Geometry check sheet. Reference: the model listing, model coordinates, mm. Give positions to 0.01 mm unless a question says otherwise; leave off trailing zeros. Loops run counter-clockwise (first coordinate to the right, second up) from the corner with the lowest first, then second, coordinate; pieces in that order, holes last. Notation, with made-up numbers: (79.5, -5.75) -> (117.5, -5.75) arc R35 ccw to (117.5, 26.25) -> close; hole circle Ø10 at (-1.75, -34). An arc over 180 degrees is marked (long way). Write item = value, one per line. Start each with the question number.
```python
from build123d import *

# Parameters (mm, degrees)
F1_DEPTH = 10


# Not quite as in the source:
# - a feature names something its author has since deleted; it is built from what else it names


with BuildPart() as f1:
    # F0 (on Front) → F1 (new body)
    with BuildSketch(Plane.XZ):
        with BuildLine():
            Line((-0.4689496755, 31.1130427234), (-12.4689496755, 31.1130427234))
            Line((-12.4689496755, 31.1130427234), (-12.4689496755, 20.1130427234))
            Line((-12.4689496755, 20.1130427234), (-6.4189496755, 20.1130427234))
            ThreePointArc((-6.4189496755, 20.1130427234), (-4.9689496755, 21.5630427234), (-3.5189496755, 20.1130427234))
            ThreePointArc((-3.5189496755, 20.1130427234), (-3.9436448428, 19.0877378907), (-4.9689496755, 18.6630427234))
            Line((-4.9689496755, 18.6630427234), (-4.9689496755, 13.4656252339))
            Line((-4.9689496755, 13.4656252339), (-0.4689496755, 13.4656252339))
            Line((-0.4689496755, 13.4656252339), (-0.4689496755, 31.1130427234))
        make_face()
        with BuildLine():
            Line((-12.4689496755, 31.1130427234), (-24.4689496755, 31.1130427234))
            Line((-24.4689496755, 31.1130427234), (-24.4689496755, 20.1130427234))
            Line((-24.4689496755, 20.1130427234), (-21.4189496755, 20.1130427234))
            ThreePointArc((-21.4189496755, 20.1130427234), (-19.9689496755, 21.5630427234), (-18.5189496755, 20.1130427234))
            Line((-18.5189496755, 20.1130427234), (-12.4689496755, 20.1130427234))
            Line((-12.4689496755, 20.1130427234), (-12.4689496755, 31.1130427234))
        make_face()
        with BuildLine():
            Line((-6.4189496755, 20.1130427234), (-12.4689496755, 20.1130427234))
            Line((-12.4689496755, 20.1130427234), (-18.5189496755, 20.1130427234))
            ThreePointArc((-18.5189496755, 20.1130427234), (-18.9436448428, 19.0877378907), (-19.9689496755, 18.6630427234))
            Line((-19.9689496755, 18.6630427234), (-19.9689496755, 6.5630427234))
            ThreePointArc((-19.9689496755, 6.5630427234), (-18.9436448428, 6.1383475561), (-18.5189496755, 5.1130427234))
            Line((-18.5189496755, 5.1130427234), (-6.4189496755, 5.1130427234))
            ThreePointArc((-6.4189496755, 5.1130427234), (-5.9942545082, 6.1383475561), (-4.9689496755, 6.5630427234))
            Line((-4.9689496755, 6.5630427234), (-4.9689496755, 13.4656252339))
            Line((-4.9689496755, 13.4656252339), (-4.9689496755, 18.6630427234))
            ThreePointArc((-4.9689496755, 18.6630427234), (-5.9942545082, 19.0877378907), (-6.4189496755, 20.1130427234))
        make_face()
        with BuildLine():
            Line((-21.4189496755, 20.1130427234), (-24.4689496755, 20.1130427234))
            Line((-24.4689496755, 20.1130427234), (-24.4689496755, -0.8869572766))
            Line((-24.4689496755, -0.8869572766), (-0.4689496755, -0.8869572766))
            Line((-0.4689496755, -0.8869572766), (-0.4689496755, 13.4656252339))
            Line((-0.4689496755, 13.4656252339), (-4.9689496755, 13.4656252339))
            Line((-4.9689496755, 13.4656252339), (-4.9689496755, 6.5630427234))
            ThreePointArc((-4.9689496755, 6.5630427234), (-3.9436448428, 6.1383475561), (-3.5189496755, 5.1130427234))
            ThreePointArc((-3.5189496755, 5.1130427234), (-4.9689496755, 3.6630427234), (-6.4189496755, 5.1130427234))
            Line((-6.4189496755, 5.1130427234), (-18.5189496755, 5.1130427234))
            ThreePointArc((-18.5189496755, 5.1130427234), (-20.9942545082, 4.0877378907), (-19.9689496755, 6.5630427234))
            Line((-19.9689496755, 6.5630427234), (-19.9689496755, 18.6630427234))
            ThreePointArc((-19.9689496755, 18.6630427234), (-20.9942545082, 19.0877378907), (-21.4189496755, 20.1130427234))
        make_face()
    extrude(amount=F1_DEPTH)


solid = f1.part
```
1) Section check B-B (z = 19.5). Enter the section's corners in (x, y), plus the area to 3 significant figures.
2) Thickness scan on line 1 (X direction, y = -1, z = 5); line 2 (Z direction, x = -20.5, y = -6.75); line 3 (X direction, y = -5.75, z = 4). Record the ranges inside material, lowest first.
3) Section check A-A (y = -3). Enter the section's corners in (x, z), plus the area to 3 significant figures.
4) Section check C-C (x = -4). Enter the section's corners in (y, z).
Check result:
q1.outline = (-24.47, -10) -> (-21.28, -10) -> (-21.28, 0) -> (-24.47, 0) -> close; (-18.65, -10) -> (-6.28, -10) -> (-6.28, 0) -> (-18.65, 0) -> close; (-3.65, -10) -> (-0.47, -10) -> (-0.47, 0) -> (-3.65, 0) -> close
q1.area = 187 mm2
q2.line_1 = -24.47 to -21.41, -18.52 to -6.41, -3.52 to -0.47
q2.line_2 = -0.89 to 3.76, 6.46 to 18.76, 21.46 to 31.11
q2.line_3 = -24.47 to -20.9, -19.04 to -5.9, -4.04 to -0.47
q3.outline = (-24.47, -0.89) -> (-0.47, -0.89) -> (-0.47, 31.11) -> (-24.47, 31.11) -> close; hole circle Ø2.9 at (-19.97, 5.11); hole circle Ø2.9 at (-19.97, 20.11); hole circle Ø2.9 at (-4.97, 5.11); hole circle Ø2.9 at (-4.97, 20.11)
q3.area = 742 mm2
q4.outline = (-10, -0.89) -> (0, -0.89) -> (0, 4.03) -> (-10, 4.03) -> close; (-10, 6.19) -> (0, 6.19) -> (0, 19.03) -> (-10, 19.03) -> close; (-10, 21.19) -> (0, 21.19) -> (0, 31.11) -> (-10, 31.11) -> close
